Work out the finished part from the listing and answer in its coordinate system (mm). A direction names the side the tool comes from. Round coordinates to 2 decimals unless told otherwise and drop trailing zeros. Order: outer loops, then holes, each group sorted by start corner. A loop starts at its lowest first (then second) coordinate and runs counter-clockwise, first axis right, second up. Notation, with made-up numbers: (67, -21) -> (83, -21) arc R33 ccw to (83, 17) -> close; hole circle Ø6 at (-5, -17.75). An arc over 180 degrees is marked (long way). Use a Markdown table: item, result. Add a question column.
Item 1: A tool of negligible diameter and unlimited length cuts with its end or side. For faces 4 (the cylindrical face through (-1.926, 18.961, -0.607)), 5 (the flat face through (-1, 0, -2)), 6 (the cylindrical face through (3.267, 6.439, -1.699)), from which of +Z, -Z, +X, -X, +Y, -Y can it reach the whole face along a straight path? Write none if from no direction.
Item 2: Find the intervals of material crossed by L1, parallel to X at y = 6.75, z = -1.5; L2, parallel to X at y = 8, z = -0.75, in increasing order. Write a range as [from, to].
Item 3: A cutting plane is placed at C-C, the plane y = 10.75. Determine the outline of the cut face in (x, z), plus the area to 3 significant figures.
Item 4: A cutting plane is placed at B-B, the plane z = 3. Determine the outline of the cut face in (x, y), plus the area to 3 significant figures.
Item 5: A cutting plane is placed at D-D, the plane x = -2.5. Determine the outline of the cut face in (y, z), plus the area to 3 significant figures.
Item 6: For a pull along Z with two mould halves and no side action, classify faces 1 (the cylindrical face through (3.874, 19.139, 0.86)), 2 (the cylindrical face through (1.8, 6.4, -0.6)), 3 (the flat face through (-1, 25.4, 2)) as +Z half, -Z half, draft (parallel to the pull), parting line (faces both ways), or undercut.
Item 7: Flat-ended cylindrical pins translate along their axes: P1, Ø3, axis at x = -2.5, y = 20.5, coming from the +Z side; P2, Ø4, axis at x = 3, y = 11.5, coming from the -Z side. Find the tip coordinate at first contact, or state that the pin passes through.
Item 8: A cutting plane is placed at A-A, the plane x = 0. Determine the outline of the cut face in (y, z).
from build123d import *

# Parameters (mm, degrees)
F_10_32_TAPPED_HOLE1_D     = 4.0386
F_10_32_TAPPED_HOLE1_DEPTH = 12.7
F_10_32_TAPPED_HOLE1_TIP   = 1.213317848
F_10_24_TAPPED_HOLE1_D     = 3.7973
F_10_24_TAPPED_HOLE1_DEPTH = 15.24
F_10_24_TAPPED_HOLE1_TIP   = 1.140824014


with BuildPart() as part:
    # Sketch1 → Revolve1 (revolve)
    with BuildSketch(Plane.XY, mode=Mode.PRIVATE) as revolve1_sk:
        Polygon((0, 0), (3.683, 0), (3.683, 12.7), (3.96875, 12.7), (3.96875, 25.4), (0, 25.4), align=None)
    revolve(revolve1_sk.sketch.rotate(Axis((0, 0, 0), (0, 1, 0)), 90), axis=Axis((0, 0, 0), (0, 1, 0)))

    # #10-32 Tapped Hole1
    with Locations(Plane(origin=(0, 25.4, 0), x_dir=(1, 0, 0), z_dir=(0, 1, 0))):
        with Locations((0, 0)):
            Hole(F_10_32_TAPPED_HOLE1_D / 2, depth=F_10_32_TAPPED_HOLE1_DEPTH)
            with Locations((0, 0, -(F_10_32_TAPPED_HOLE1_DEPTH + F_10_32_TAPPED_HOLE1_TIP / 2))):  # 118° drill point
                Cone(0, F_10_32_TAPPED_HOLE1_D / 2, F_10_32_TAPPED_HOLE1_TIP, mode=Mode.SUBTRACT)

    # #10-24 Tapped Hole1
    with Locations(Plane(origin=(0, 0, 0), x_dir=(-1, 0, 0), z_dir=(0, -1, 0))):
        with Locations((0, 0)):
            Hole(F_10_24_TAPPED_HOLE1_D / 2, depth=F_10_24_TAPPED_HOLE1_DEPTH)
            with Locations((0, 0, -(F_10_24_TAPPED_HOLE1_DEPTH + F_10_24_TAPPED_HOLE1_TIP / 2))):  # 118° drill point
                Cone(0, F_10_24_TAPPED_HOLE1_D / 2, F_10_24_TAPPED_HOLE1_TIP, mode=Mode.SUBTRACT)


solid = part.part
Reported:
| question | item | result |
|---|---|---|
| 1 | face 4 | +Y |
| 1 | face 5 | +Z, -Z, +X, -X, -Y |
| 1 | face 6 | -Y |
| 2 | L1 | [-3.36, -1.16], [1.16, 3.36] |
| 2 | L2 | [-3.61, -1.74], [1.74, 3.61] |
| 3 | outline | circle Ø7.37 at (0, 0); hole circle Ø3.8 at (0, 0) |
| 3 | area | 31.3 mm² |
| 4 | outline | (-2.6, 12.7) -> (-2.14, 12.7) -> (-2.14, 0) -> (2.14, 0) -> (2.14, 12.7) -> (2.6, 12.7) -> (2.6, 25.4) -> (-2.6, 25.4) -> close |
| 4 | area | 120 mm² |
| 5 | outline | (0, -2.7) -> (12.7, -2.7) -> (12.7, -3.08) -> (25.4, -3.08) -> (25.4, 3.08) -> (12.7, 3.08) -> (12.7, 2.7) -> (0, 2.7) -> close |
| 5 | area | 147 mm² |
| 6 | face 1 | parting line |
| 6 | face 2 | undercut |
| 6 | face 3 | draft |
| 7 | P1 | z = 3.84 |
| 7 | P2 | z = -3.71 |
| 8 | outline | (0, -3.68) -> (12.7, -3.68) -> (12.7, -3.97) -> (25.4, -3.97) -> (25.4, -2.02) -> (12.7, -2.02) -> (12.63, -1.9) -> (0, -1.9) -> close; (0, 1.9) -> (12.63, 1.9) -> (12.7, 2.02) -> (25.4, 2.02) -> (25.4, 3.97) -> (12.7, 3.97) -> (12.7, 3.68) -> (0, 3.68) -> close |
